from build123d import *

# Parameters (mm, degrees)
SKETCH_R        = 3
PAD_DEPTH       = 6.5
SKETCH001_R     = 6.1
SKETCH001_R_2   = 3
PAD001_DEPTH    = 10
PAD002_DEPTH    = 13
SKETCH003_R     = 6.1
POCKET_DEPTH    = 6
POCKET001_DEPTH = 5
SKETCH005_R     = 1.6
POCKET002_DEPTH = 17.001
SKETCH006_R     = 1.6
POCKET003_DEPTH = 21.251


with BuildPart() as part:
    # Sketch → Pad (new body)
    with BuildSketch(Plane.XY):
        Polygon((9.814955, 0), (4.907477, 8.5), (-4.907477, 8.5), (-9.814955, 0), (-4.907477, -8.5), (4.907477, -8.5), align=None)
        Circle(SKETCH_R, mode=Mode.SUBTRACT)
    extrude(amount=PAD_DEPTH)

    # Sketch001 (on Face9 of Pad) → Pad001 (join)
    with BuildSketch(Plane.XY.offset(6.5)):
        Circle(SKETCH001_R)
        Circle(SKETCH001_R_2, mode=Mode.SUBTRACT)
    extrude(amount=PAD001_DEPTH)

    # Sketch002 (on Face12 of Pad001) → Pad002 (join)
    with BuildSketch(Plane.XY.offset(16.5)):
        with BuildLine():
            Line((-1.658312, 2.5), (1.658312, 2.5))
            ThreePointArc((1.658312, 2.5), (0, 3), (-1.658312, 2.5))
        make_face()
    extrude(amount=-PAD002_DEPTH)

    # Sketch003 (on Face15 of Pad002) → Pocket (cut)
    with BuildSketch(Plane.XY.offset(16.5)):
        Circle(SKETCH003_R)
    extrude(amount=-POCKET_DEPTH, mode=Mode.SUBTRACT)

    # Sketch004 (on Face4 of Pocket) → Pocket001 (cut)
    with BuildSketch(Plane(origin=(0, 0, 0), x_dir=(1, 0, 0), z_dir=(0, 0, -1))):
        Polygon((2.886751, 5), (-2.886751, 5), (-5.773503, 0), (-2.886751, -5), (2.886751, -5), (5.773503, 0), align=None)
    extrude(amount=-POCKET001_DEPTH, mode=Mode.SUBTRACT)

    # Sketch005 (on Face6 of Pocket001) → Pocket002 (cut, through all)
    with BuildSketch(Plane.XZ.offset(8.5)):
        with Locations((0, 2.5)):
            Circle(SKETCH005_R)
    extrude(amount=-POCKET002_DEPTH, mode=Mode.SUBTRACT)

    # Sketch006 → Pocket003 (cut, through all)
    with BuildSketch(Plane(origin=(7.361216, 4.25, 0), x_dir=(-0.5, 0.866025, 0), z_dir=(0.866025, 0.5, 0))):
        with Locations((0, 2.5)):
            Circle(SKETCH006_R)
    extrude(amount=-POCKET003_DEPTH, mode=Mode.SUBTRACT)


solid = part.part
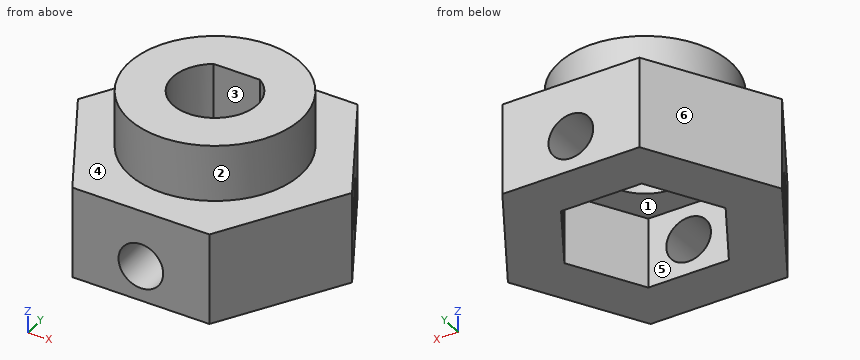
CAD build for the part. Positions are in the model's coordinates, mm. Face numbers are marked on the shaded views. A direction names the side the tool comes from. Round coordinates to 2 decimals unless told otherwise and drop trailing zeros. Order: outer loops, then holes, each group sorted by start corner. A loop starts at its lowest first (then second) coordinate and runs counter-clockwise, first axis right, second up. Notation, with made-up numbers: (15.25, 73) -> (32.25, 73) arc R25 cw to (32.25, 98) -> close; hole circle Ø10 at (75.25, 65). An arc over 180 degrees is marked (long way). Write each question's results on one line, items separated by ' | '.
1. Cut at B-B (z = 2.5). Give the cut face in (x, y), plus the area to 3 significant figures.
Findings below:
outline: (-9.81, 0) -> (-8.16, -2.86) -> (-5.13, -1.11) -> (-5.77, 0) -> (-2.89, 5) -> (-1.6, 5) -> (-1.6, 8.5) -> (-4.91, 8.5) -> close; (-6.56, -5.64) -> (-4.91, -8.5) -> (-1.6, -8.5) -> (-1.6, -5) -> (-2.89, -5) -> (-3.53, -3.89) -> close; (1.6, -8.5) -> (4.91, -8.5) -> (9.81, 0) -> (8.16, 2.86) -> (5.13, 1.11) -> (5.77, 0) -> (2.89, -5) -> (1.6, -5) -> close; (1.6, 5) -> (2.89, 5) -> (3.53, 3.89) -> (6.56, 5.64) -> (4.91, 8.5) -> (1.6, 8.5) -> close | area: 119 mm²
2. Cut at A-A (x = 0). Give the cut face in (y, z).
Findings below:
outline: (-8.5, 0) -> (-5, 0) -> (-5, 0.9) -> (-8.5, 0.9) -> close; (-8.5, 4.1) -> (-5, 4.1) -> (-5, 5) -> (-3, 5) -> (-3, 10.5) -> (-6.1, 10.5) -> (-6.1, 6.5) -> (-8.5, 6.5) -> close; (2.5, 5) -> (5, 5) -> (5, 4.1) -> (8.5, 4.1) -> (8.5, 6.5) -> (6.1, 6.5) -> (6.1, 10.5) -> (2.5, 10.5) -> close; (5, 0) -> (8.5, 0) -> (8.5, 0.9) -> (5, 0.9) -> close
3. 3-axis set-ups, long thin cutter, end or side, ignore diameter. For the marked faces 1, 2 and 3: which of +Z, -Z, +X, -X, +Y, -Y reach the whole face in a straight line?
Findings below:
face 1: -Z | face 2: +Z | face 3: +Z, -Z
4. Pull direction X, two halves, no side cores. Call the marked faces 4, 5 and 6: pulls with the +X half, pulls with the -X half, needs draft (parallel to the pull), parting line crosses it, or undercut.
Findings below:
face 4: needs draft | face 5: undercut | face 6: pulls with the -X half
5. Wall check: line 1 along Z through (x, y) = (0, 5.85); line 2 along Y through (x, z) = (0, 7.75); line 3 along Z through (x, y) = (0, 7.3). Give the ranges that are in metal, low to high. Write a range as [from, to].
Findings below:
line 1: z = [0, 0.9], [4.1, 10.5] | line 2: y = [-6.1, -3], [2.5, 6.1] | line 3: z = [0, 0.9], [4.1, 6.5]
6. Cut at C-C (y = 6.75). Give the cut face in (x, z), plus the area to 3 significant figures.
Findings below:
outline: (-5.92, 0) -> (5.92, 0) -> (5.92, 6.5) -> (-5.92, 6.5) -> close; hole circle Ø3.2 at (0, 2.5) | area: 68.9 mm²
7. Flat gauge pins, fed straight in: P1, Ø3, axis at y = 5, z = 3.5, coming from the -X side; P2, Ø3, axis at x = 2.5, y = -1.5, coming from the -Z side; P3, Ø1.7, axis at x = -0.5, z = 7.5, coming from the -Y side. Where does each tip first touch, or does it go through?
Findings below:
P1: stops at x = -7.79 | P2: stops at z = 5 | P3: stops at y = -6.1
8. Cut at D-D (z = 8). Give the cut face in (x, y).
Findings below:
outline: circle Ø12.2 at (0, 0); hole (-1.66, 2.5) arc R3 ccw (long way) to (1.66, 2.5) -> close
